Geometry check sheet. Reference: the model listing, model coordinates, mm. A direction names the side the tool comes from. Coordinates: 2 decimals unless noted, no trailing zeros. Loops run counter-clockwise (first coordinate to the right, second up) from the corner with the lowest first, then second, coordinate; pieces in that order, holes last. Notation, with made-up numbers: M 67,31.5 L 82,31.5 A30 cw 82,54.5 Z; hole C 47.5,-25.5 d4. An arc over 180 degrees is marked long. One line per question, with ' | ' between items. Start each with the question number.
from build123d import *

# Parameters (mm, degrees)
SKETCH1_R           = 3.000027903
BOSS_EXTRUDE1_DEPTH = 4
BOSS_EXTRUDE4_DEPTH = 3.5
BOSS_EXTRUDE6_DEPTH = 34
BOSS_EXTRUDE7_DEPTH = 3.5
SKETCH8_R           = 3.000027903
BOSS_EXTRUDE8_DEPTH = 4


with BuildPart() as part:
    # Sketch1 → Boss-Extrude1 (new body)
    with BuildSketch(Plane.XY):
        with BuildLine():
            ThreePointArc((-35.515, 3.29389), (-36.500003461, -2e-06), (-35.515, -3.293894))
            add(Edge.make_bspline(
                [(-35.515, -3.293894), (-34.604438991, -5.156956918), (-33.54048, -6.937562)],
                knots=[0, 0, 0, 1, 1, 1], degree=2))
            ThreePointArc((-33.54048, -6.937562), (-30.745960827, -9.193764608), (-27.245993386, -10.000000017))
            Line((-27.245993386, -10.000000017), (-16.999993386, -10.000000017))
            Line((-16.999993386, -10.000000017), (-16.999993386, 9.999999983))
            Line((-16.999993386, 9.999999983), (-27.245993386, 9.999999983))
            ThreePointArc((-27.245993386, 9.999999983), (-31.011968955, 9.057189861), (-33.875915, 6.4362595))
            add(Edge.make_bspline(
                [(-33.875915, 6.4362595), (-34.671605619, 4.852572547), (-35.515, 3.29389)],
                knots=[0, 0, 0, 1, 1, 1], degree=2))
        make_face()
        with Locations((-30.500046711, -2e-06)):
            Circle(SKETCH1_R, mode=Mode.SUBTRACT)
    extrude(amount=BOSS_EXTRUDE1_DEPTH)

    # Sketch5 → Boss-Extrude4 (add)
    with BuildSketch(Plane(origin=(-16.999993386, 0, 0), x_dir=(0, 0, -1), z_dir=(1, 0, 0))):
        with BuildLine():
            Line((4.999999299, 2.000001386), (0, 2.000001386))
            Line((0, 2.000001386), (0, -10.000000017))
            Line((0, -10.000000017), (4.999999299, -10.000000017))
            ThreePointArc((4.999999299, -10.000000017), (9.242640482, -8.242640499), (11, -3.999999316))
            ThreePointArc((11, -3.999999316), (9.242640482, 0.242641867), (4.999999299, 2.000001386))
        make_face()
        with BuildLine():
            ThreePointArc((5.745163587, -1.412519358), (7.746056235, -2.073529521), (8.6, -3.999999316))
            ThreePointArc((8.6, -3.999999316), (8.009825654, -5.649423344), (6.507230229, -6.550041118))
            ThreePointArc((6.507230229, -6.550041118), (3.428142195, -4.381492167), (5.745163587, -1.412519358))
        make_face(mode=Mode.SUBTRACT)
    extrude(amount=-BOSS_EXTRUDE4_DEPTH)

    # Sketch5<4> → Boss-Extrude6 (add)
    with BuildSketch(Plane(origin=(-16.999993386, 0, 0), x_dir=(0, 0, -1), z_dir=(1, 0, 0))):
        Polygon((-2, -2.292812017), (-3.500601, 9.999999983), (-4, 9.999999983), (-4, -10.000000017), (-2, -10.000000017), align=None)
    extrude(amount=BOSS_EXTRUDE6_DEPTH)



with BuildPart() as body_2:
    # Sketch7 → Boss-Extrude7 (new body)
    with BuildSketch(Plane(origin=(17.000006614, 0, 0), x_dir=(0, 0, -1), z_dir=(1, 0, 0))):
        with BuildLine():
            Line((4.999999299, 1.98580143), (0, 1.98580143))
            Line((0, 1.98580143), (0, -10.014199973))
            Line((0, -10.014199973), (4.999999299, -10.014199973))
            ThreePointArc((4.999999299, -10.014199973), (9.242640482, -8.256840455), (11, -4.014199272))
            ThreePointArc((11, -4.014199272), (9.242640482, 0.228441911), (4.999999299, 1.98580143))
        make_face()
        with BuildLine():
            ThreePointArc((5.745163587, -1.426719314), (7.746056235, -2.087729477), (8.6, -4.014199272))
            ThreePointArc((8.6, -4.014199272), (8.009825654, -5.6636233), (6.507230229, -6.564241074))
            ThreePointArc((6.507230229, -6.564241074), (3.428142195, -4.395692123), (5.745163587, -1.426719314))
        make_face(mode=Mode.SUBTRACT)
    extrude(amount=BOSS_EXTRUDE7_DEPTH)


with BuildPart() as part_1:
    add(part.part)

    add(body_2.part)  # Boss-Extrude8 merges body 2
    # Sketch8 → Boss-Extrude8 (add)
    with BuildSketch(Plane.XY.offset(4)):
        with BuildLine():
            Line((17.000006614, -10.000000017), (27.246006614, -9.904922539))
            ThreePointArc((27.246006614, -9.904922539), (31.344343382, -9.110808917), (34.467826641, -6.341182039))
            add(Edge.make_bspline(
                [(34.467826641, -6.341182039), (35.26351726, -4.757495086), (36.106911641, -3.198812539)],
                knots=[0, 0, 0, 1, 1, 1], degree=2))
            ThreePointArc((36.106911641, -3.198812539), (37.091915102, 0.095079461), (36.106911641, 3.388971461))
            add(Edge.make_bspline(
                [(36.106911641, 3.388971461), (35.255873472, 5.530984122), (33.464737791, 7.032639461)],
                knots=[0, 0, 0, 1, 1, 1], degree=2))
            ThreePointArc((33.464737791, 7.032639461), (30.691215095, 9.22014949), (27.246006614, 9.999999983))
            Line((27.246006614, 9.999999983), (17.000006614, 9.999999983))
            Line((17.000006614, 9.999999983), (17.000006614, -8.622062624))
            Line((17.000006614, -8.622062624), (17.000006614, -10.000000017))
        make_face()
        with Locations((31.091958352, 0.095079461)):
            Circle(SKETCH8_R, mode=Mode.SUBTRACT)
    extrude(amount=-BOSS_EXTRUDE8_DEPTH)


solid = part_1.part
1. Sectioned sample at A-A (z = -10). Record the cut outline in (x, y), and give its area (3 significant figures).
2. Sectioned sample at C-C (z = 1). State how many separate pieces and enclosed holes the cut face has, and give its area (3 significant figures).
3. Tool access check on faces 1 (the flat face through (-27, 0, 0)), 2 (the cylindrical face through (30.736, 9.199, 2.028)), 3 (the flat face through (-20.5, -4, -3)), 4 (the flat face through (20.5, -4, -3)), 5 (the flat face through (-19, 2, -3)). Record the directions out of +Z, -Z, +X, -X, +Y, -Y that give a thin tool (end or side, any length) a straight path to the whole face; none if there is none.
4. Depth check by flat-ended pin: pin 1 Ø8 at (x, y) = (-30.5, 0) entering from -Z; pin 2 Ø9 at (y, z) = (-4, -5.5) entering from +X; pin 3 Ø6 at (x, y) = (1, 7.5) entering from -Z; pin 4 Ø3 at (y, z) = (6, -2.5) entering from -X. Enter the tip coordinate at first touch or a pass-through.
5. Sectioned sample at B-B (x = -10.5). Record the cut outline in (y, z), and give its area (3 significant figures).
6. Thickness scan on line 1 (X direction, y = -5.75, z = -9.25); line 2 (Z direction, x = -24, y = -2); line 3 (Y direction, x = -26.5, z = 2.5). Record the ranges inside material, lowest first.
7. Draft check along Y on faces 6 (the cylindrical face through (37.09, 0.05, 2.03)), 7 (the flat face through (27, 0, 0)), 8 (the cylindrical face through (-33.5, 0.1, 2)), 9 (the cylindrical face through (31.291, -9.137, 2.028)). Enter one of: +Y half, -Y half, draft (parallel to the pull), parting line (faces both ways), or undercut.
Result:
1) outline: M -20.5,-7.32 L -17,-7.32 L -17,-0.68 L -20.5,-0.68 Z; M 17,-7.33 L 20.5,-7.33 L 20.5,-0.7 L 17,-0.7 Z | area: 46.4 mm2
2) separate pieces: 2 | enclosed holes: 2 | area: 640 mm2
3) face 1: -Z, -X, +Y | face 2: +Z, -Z, +X, +Y | face 3: -Z, -X, +Y, -Y | face 4: -Z, +X, +Y, -Y | face 5: -Z, +X, -X, +Y
4) pin 1: stops at z = 0 | pin 2: stops at x = 20.5 | pin 3: stops at z = 2.83 | pin 4: passes through
5) outline: M -10,2 L -2.29,2 L 10,3.5 L 10,4 L -10,4 Z | area: 30.8 mm2
6) line 1: x = -20.5 to -17, 17 to 20.5 | line 2: z = 0 to 4 | line 3: y = -10 to 10
7) face 6: parting line | face 7: draft | face 8: undercut | face 9: -Y half
